Can you work these out from the model? Positions are in its coordinate system, mm. A direction names the side the tool comes from. Coordinates: 2 decimals unless noted, no trailing zeros. Order: outer loops, then holes, each group sorted by start corner. A loop starts at its lowest first (then second) coordinate and runs counter-clockwise, first axis right, second up. Notation, with made-up numbers: (73, -36) -> (129, -36) arc R31 cw to (129, -8) -> close; hole circle Ø11 at (-18, 58.5). An arc over 180 degrees is marked (long way). Answer in a Markdown table with one row per item. Add a question column.
1. On a 3-axis mill with a long thin cutter (end or side, diameter ignored), from which of +Z, -Z, +X, -X, +Y, -Y can I reach the whole of each face in a straight line? I mean faces 1 (the face through (-10.711, -0.986, -31.629)), 2 (the face through (-27.14, 2.54, -23.39)), 3 (the face through (3, 0, 24.75)), 4 (the face through (-36, 0, 0)). Say none if no direction works.
2. We'd pull the mould along Y, two halves only. Please class faces 5 (the face through (-22.495, -0.07, 0.495)), 6 (the face through (-23, 0, 25)), 7 (the face through (-5, -3.5, -29)): pulls with the +Y half, pulls with the -Y half, needs draft (parallel to the pull), parting line crosses it, or undercut.
3. Imagine slicing it at B-B on x = 1.5. Write out the boundary of the cut face in (y, z), plus the area to 3 significant figures.
4. Imagine slicing it at D-D on z = 0. Write out the boundary of the cut face in (x, y), plus the area to 3 significant figures.
5. Imagine slicing it at C-C on y = 1.5. State how many separate pieces and enclosed holes the cut face has, plus the area to 3 significant figures.
6. Will these pins go through, and if not, where does the flat tip stop? pin 1 (4.5 mm diameter, centred on y = 0, z = 29.25, fed in from -X); pin 2 (10 mm diameter, centred on x = -3.5, z = -20, fed in from +Y); pin 3 (5 mm diameter, centred on y = -2, z = -26, fed in from +X); pin 4 (3.5 mm diameter, centred on x = -25.5, y = 1.5, fed in from -Z).
7. If I drill on line 1 along Z through (x, y) = (-6, 3.25); line 2 along Z through (x, y) = (-8.5, 0.5); line 3 along Z through (x, y) = (2.5, 2.5), over which ranges is the centre line in solid material (lowest first)? Write a range as [from, to].
8. Imagine slicing it at A-A on z = -29.25. Write out the boundary of the cut face in (x, y) (3 decimals).
from build123d import *

# Parameters (mm, degrees)
BOSS_EXTRUDE1_DEPTH      = 5
BOSS_EXTRUDE1_DEPTH_BACK = 5
SKETCH1_R                = 1.5
CUT_EXTRUDE1_DEPTH       = 5
BOSS_EXTRUDE2_DEPTH      = 3.5
BOSS_EXTRUDE2_DEPTH_BACK = 3.5
SKETCH3_W                = 7
SKETCH3_H                = 9
CUT_EXTRUDE2_DEPTH       = 3.5
CUT_EXTRUDE2_DEPTH_BACK  = 3.5
SKETCH4_W                = 9.454278837
SKETCH4_H                = 9.5
SKETCH5_R                = 2.575
CUT_EXTRUDE3_DEPTH       = 2.55
SKETCH6_R                = 2.575
CUT_EXTRUDE4_DEPTH       = 2.55


with BuildPart() as part:
    # Sketch1 → Boss-Extrude1 (new, two sides: drawn at the far end of the back side and taken through both)
    with BuildSketch(Plane(origin=(0, 0, 0), x_dir=(1, 0, 0), z_dir=(0, 1, 0)).offset(-BOSS_EXTRUDE1_DEPTH_BACK)):
        with BuildLine():
            Line((0, 22.5), (0, 36))
            Line((0, 36), (-18.553975315, 36))
            ThreePointArc((-18.553975315, 36), (-28.637824638, 28.637824638), (-36, 18.553975315))
            Line((-36, 18.553975315), (-36, -18.553975315))
            ThreePointArc((-36, -18.553975315), (-28.637824638, -28.637824638), (-18.553975315, -36))
            Line((-18.553975315, -36), (0, -36))
            Line((0, -36), (0, -22.5))
            ThreePointArc((0, -22.5), (-22.5, 0), (0, 22.5))
        make_face()
        with Locations(Location((-24.748737342, -24.748737342, 0), (0, 0, 270))):
            Circle(SKETCH1_R, mode=Mode.SUBTRACT)
        with Locations(Location((-24.748737342, 24.748737342, 0), (0, 0, 270))):
            Circle(SKETCH1_R, mode=Mode.SUBTRACT)
    extrude(amount=BOSS_EXTRUDE1_DEPTH + BOSS_EXTRUDE1_DEPTH_BACK)

    # Sketch2 → Cut-Extrude1 (cut)
    with BuildSketch(Plane(origin=(0, 5, 0), x_dir=(1, 0, 0), z_dir=(0, 1, 0))):
        Polygon((-23.161024101, 27.498737342), (-26.336450582, 27.498737342), (-27.924163822, 24.748737342), (-26.336450582, 21.998737342), (-23.161024101, 21.998737342), (-21.573310861, 24.748737342), align=None)
    cut_extrude1 = extrude(amount=-CUT_EXTRUDE1_DEPTH, mode=Mode.SUBTRACT)

    # Mirror1: Cut-Extrude1 across plane
    add(cut_extrude1.mirror(Plane.XY), mode=Mode.SUBTRACT)

    # Sketch3 → Boss-Extrude2 (add, two sides: drawn at the far end of the back side and taken through both)
    with BuildSketch(Plane(origin=(0, 0, 0), x_dir=(1, 0, 0), z_dir=(0, 1, 0)).offset(-BOSS_EXTRUDE2_DEPTH_BACK)):
        with Locations((3.5, -29.25)):
            Rectangle(SKETCH3_W, SKETCH3_H)
    extrude(amount=BOSS_EXTRUDE2_DEPTH + BOSS_EXTRUDE2_DEPTH_BACK)

    # Sketch4 → Cut-Extrude2 (cut, two sides: drawn at the far end of the back side and taken through both)
    with BuildSketch(Plane.XZ.offset(-CUT_EXTRUDE2_DEPTH_BACK)):
        with Locations((-4.727139419, -29.25)):
            Rectangle(SKETCH4_W, SKETCH4_H)
    extrude(amount=CUT_EXTRUDE2_DEPTH + CUT_EXTRUDE2_DEPTH_BACK, mode=Mode.SUBTRACT)

    # Sketch5 → Cut-Extrude3 (cut)
    with BuildSketch(Plane(origin=(7, 0, 0), x_dir=(0, 0, -1), z_dir=(1, 0, 0))):
        with Locations((-29.25, 0)):
            Circle(SKETCH5_R)
    extrude(amount=-CUT_EXTRUDE3_DEPTH, mode=Mode.SUBTRACT)

    # Sketch6 → Cut-Extrude4 (cut)
    with BuildSketch(Plane(origin=(-9.454278837, 0, 0), x_dir=(0, 0, -1), z_dir=(1, 0, 0))):
        with Locations((29.25, 0)):
            Circle(SKETCH6_R)
    extrude(amount=-CUT_EXTRUDE4_DEPTH, mode=Mode.SUBTRACT)


solid = part.part
Answers follow:
| question | item | result |
|---|---|---|
| 1 | face 1 | +X |
| 1 | face 2 | +Y |
| 1 | face 3 | -Z, +X, +Y, -Y |
| 1 | face 4 | +Z, -Z, -X, +Y, -Y |
| 2 | face 5 | needs draft |
| 2 | face 6 | pulls with the +Y half |
| 2 | face 7 | undercut |
| 3 | outline | (-3.5, 24.75) -> (3.5, 24.75) -> (3.5, 33.75) -> (-3.5, 33.75) -> close |
| 3 | area | 63.0 mm² |
| 4 | outline | (-36, -5) -> (-22.5, -5) -> (-22.5, 5) -> (-36, 5) -> close |
| 4 | area | 135 mm² |
| 5 | separate pieces | 1 |
| 5 | enclosed holes | 2 |
| 5 | area | 1,460 mm² |
| 6 | pin 1 | stops at x = -30.19 |
| 6 | pin 2 | stops at y = 5 |
| 6 | pin 3 | stops at x = 0 |
| 6 | pin 4 | stops at z = -32.81 |
| 7 | line 1 | z = [-36, -34], [-24.5, -21.69], [21.69, 36] |
| 7 | line 2 | z = [-36, -34], [-24.5, -20.83], [20.83, 36] |
| 7 | line 3 | z = [24.75, 33.75] |
| 8 | outline | (-28.012, -5) -> (0, -5) -> (0, -3.5) -> (-9.454, -3.5) -> (-9.454, -2.575) -> (-12.004, -2.575) -> (-12.004, 2.575) -> (-9.454, 2.575) -> (-9.454, 3.5) -> (0, 3.5) -> (0, 5) -> (-28.012, 5) -> close |
